Autodesk Inventor part; units mm, degrees
ref_plane "YZ Plane" through (0, 0, 0) normal (1, 0, 0) x (0, 1, 0)
ref_plane "XZ Plane" through (0, 0, 0) normal (0, 1, 0) x (-1, 0, 0)
ref_plane "XY Plane" through (0, 0, 0) normal (0, 0, 1) x (1, 0, 0)
sketch "Sketch1" plane through (0, 0, 0) normal (0, 0, 1) x (1, 0, 0)
  line L0 (0, 0) -> (0, 41.5)
  line L1 (0, 41.5) -> (2.35, 41.5)
  line L2 (2.35, 41.5) -> (2.35, 37.5)
  line L3 (2.35, 37.5) -> (4, 37.5)
  line L4 (4, 37.5) -> (4, 4)
  line L5 (4, 4) -> (2.35, 4)
  line L6 (2.35, 4) -> (2.35, 0)
  line L7 (2.35, 0) -> (0, 0)
  dimension "d0" = 33.5
  dimension "d1" = 8
  dimension "d2" = 4.7
  dimension "d3" = 4
  dimension "d4" = 4
revolve "Revolution1" add sketch "Sketch1" angle 360 about axis through (0, 0, 0) along (0, 1, 0)
properties part number "Pok Mk3 Support" material "ABS Plastic"
Model file for the job. Use its own axes, mm. A direction names the side the tool comes from. Coordinates: 2 decimals unless noted, no trailing zeros. Order: outer loops, then holes, each group sorted by start corner. A loop starts at its lowest first (then second) coordinate and runs counter-clockwise, first axis right, second up. Notation, with made-up numbers: (71, 77.25) - (80, 77.25) arc R6 cw to (80, 88.25) - close; hole circle Ø9 at (50, -11.5). An arc over 180 degrees is marked (long way). Return JSON: item names as keys, results as strings. Group by question number.
1) Saw through at C-C, the plane y = 36. Write the cut outline in (x, z).
2) Saw through at A-A, the plane z = 0. Write the cut outline in (x, y), plus the area to 3 significant figures.
3) Saw through at B-B, the plane x = 0. Write the cut outline in (y, z), plus the area to 3 significant figures.
4) Tool access for faces 1 (the flat face through (2, 37.5, 2)), 2 (the flat face through (2, 4, 2)), 3 (the cylindrical face through (-0.867, 20.516, -3.905)): list every direction of +Z, -Z, +X, -X, +Y, -Y with a clear straight run to the whole face (end or side of a thin tool).
5) Probe line 1 (Y direction, x = 0.25, z = -2.75); line 2 (X direction, y = 12, z = -2.25); line 3 (X direction, y = 35.5, z = 1.5). List the from-to ranges inside material, lowest first. Write a range as from..to.
6) Saw through at D-D, the plane y = 3. Write the cut outline in (x, z).
Values found:
{
 "1": {"outline": "circle Ø8 at (0, 0)"},
 "2": {"outline": "(-4, 4) - (-2.35, 4) - (-2.35, 0) - (2.35, 0) - (2.35, 4) - (4, 4) - (4, 37.5) - (2.35, 37.5) - (2.35, 41.5) - (-2.35, 41.5) - (-2.35, 37.5) - (-4, 37.5) - close", "area": "306 mm²"},
 "3": {"outline": "(0, -2.35) - (4, -2.35) - (4, -4) - (37.5, -4) - (37.5, -2.35) - (41.5, -2.35) - (41.5, 2.35) - (37.5, 2.35) - (37.5, 4) - (4, 4) - (4, 2.35) - (0, 2.35) - close", "area": "306 mm²"},
 "4": {"face 1": "+Y", "face 2": "-Y", "face 3": "+Y, -Y"},
 "5": {"line 1": "y = 4..37.5", "line 2": "x = -3.31..3.31", "line 3": "x = -3.71..3.71"},
 "6": {"outline": "circle Ø4.7 at (0, 0)"}
}
